```python
from build123d import *

# Parameters (mm, degrees)
F0_W           = 177.8
F0_H           = 101.6
F1_DEPTH       = 3.81
F3_W           = 114.3
F3_H           = 4.318
F4_DEPTH       = 3.811
F5_R           = 9.525
F6_DEPTH       = 9.525
F8_W           = 177.8
F8_H           = 101.6
F8_W_2         = 170.18
F8_H_2         = 93.98
F9_DEPTH       = 7.62
F10_R          = 3.556
F11_DEPTH      = 9.526
F11_DEPTH_BACK = 3.811
F7_W           = 177.8
F7_H           = 3.175
F13_DEPTH      = 7.62
F2_R           = 3.556
F14_DEPTH      = 3.811
F12_R          = 2.667
F15_DEPTH      = 3.811


with BuildPart() as f1:
    # F0 (on Top) → F1 (new body)
    with BuildSketch(Plane.XY):
        with Locations((88.9, 50.8)):
            Rectangle(F0_W, F0_H)
    extrude(amount=F1_DEPTH)

    # F3 (on Top) → F4 (cut, through all)
    with BuildSketch(Plane.XY):
        with Locations((88.9, 88.9)):
            Rectangle(F3_W, F3_H)
        with Locations((88.9, 12.7)):
            Rectangle(F3_W, F3_H)
    extrude(amount=F4_DEPTH, mode=Mode.SUBTRACT)

    # F5 (on Top) → F6 (join)
    with BuildSketch(Plane.XY):
        with Locations((12.7, 50.8)):
            Circle(F5_R)
        with Locations((12.7, 90.805)):
            Circle(F5_R)
        with Locations((12.7, 10.795)):
            Circle(F5_R)
        with Locations((165.1, 90.805)):
            Circle(F5_R)
        with Locations((165.1, 50.8)):
            Circle(F5_R)
        with Locations((165.1, 10.795)):
            Circle(F5_R)
    extrude(amount=-F6_DEPTH)

    # F8 (on Top) → F9 (join)
    with BuildSketch(Plane.XY):
        with Locations((88.9, 50.8)):
            Rectangle(F8_W, F8_H)
        with Locations((88.9, 50.8)):
            Rectangle(F8_W_2, F8_H_2, mode=Mode.SUBTRACT)
    extrude(amount=-F9_DEPTH)

    # F10 (on Top) → F11 (cut, two sides)
    with BuildSketch(Plane.XY) as f11_sk:
        with Locations((165.1, 50.8)):
            Circle(F10_R)
        with Locations((165.1, 90.805)):
            Circle(F10_R)
        with Locations((12.7, 10.795)):
            Circle(F10_R)
        with Locations((12.7, 50.8)):
            Circle(F10_R)
        with Locations((12.7, 90.805)):
            Circle(F10_R)
        with Locations((165.1, 10.795)):
            Circle(F10_R)
    extrude(amount=-F11_DEPTH, mode=Mode.SUBTRACT)
    extrude(f11_sk.sketch, amount=F11_DEPTH_BACK, mode=Mode.SUBTRACT)

    # F7 (on Top) → F13 (join)
    with BuildSketch(Plane.XY):
        with Locations((88.9, 42.8625)):
            Rectangle(F7_W, F7_H)
        with Locations((88.9, 58.7375)):
            Rectangle(F7_W, F7_H)
    extrude(amount=-F13_DEPTH)

    # F2 (on Top) → F14 (cut, through all)
    with BuildSketch(Plane.XY):
        with Locations((22.225, 69.85)):
            Circle(F2_R)
        with Locations((22.225, 31.75)):
            Circle(F2_R)
        with Locations((155.575, 69.85)):
            Circle(F2_R)
        with Locations((155.575, 31.75)):
            Circle(F2_R)
    extrude(amount=F14_DEPTH, mode=Mode.SUBTRACT)

    # F12 (on Top) → F15 (cut, through all)
    with BuildSketch(Plane.XY):
        with Locations((31.75, 50.8)):
            Circle(F12_R)
        with Locations((88.9, 50.8)):
            Circle(F12_R)
        with Locations((146.05, 50.8)):
            Circle(F12_R)
        with Locations((9.525, 25.4)):
            Circle(F12_R)
        with Locations((9.525, 76.2)):
            Circle(F12_R)
        with Locations((168.275, 25.4)):
            Circle(F12_R)
        with Locations((168.275, 76.2)):
            Circle(F12_R)
        with Locations((69.85, 50.8)):
            Circle(F12_R)
        with Locations((107.95, 50.8)):
            Circle(F12_R)
        with Locations((50.8, 50.6974235177)):
            Circle(F12_R)
        with Locations((127, 50.6266094744)):
            Circle(F12_R)
    extrude(amount=F15_DEPTH, mode=Mode.SUBTRACT)


solid = f1.part
```
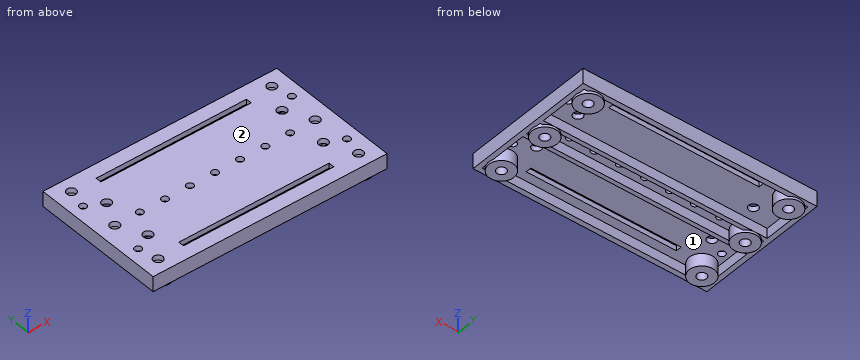
Geometry check sheet. Reference: the model listing, model coordinates, mm. Face numbers are marked on the shaded views. Coordinates: 2 decimals unless noted, no trailing zeros. Order: outer loops, then holes, each group sorted by start corner. A loop starts at its lowest first (then second) coordinate and runs counter-clockwise, first axis right, second up.
Q1. Depth check by flat-ended pin: pin 1 Ø6.5 at (x, y) = (165.1, 10.795) entering from +Z; pin 2 Ø1.5 at (x, y) = (120.5, 23) entering from -Z. Enter the tip coordinate at first touch or a pass-through.
Reply:
pin 1: passes through
pin 2: stops at z = 0
Q2. Sectioned sample at B-B on y = 69.85. Record the cut outline in (x, z), and give its area (3 significant figures).
Reply:
outline: (0, -7.62) - (3.81, -7.62) - (3.81, 0) - (18.67, 0) - (18.67, 3.81) - (0, 3.81) - close; (25.78, 0) - (152.02, 0) - (152.02, 3.81) - (25.78, 3.81) - close; (159.13, 0) - (173.99, 0) - (173.99, -7.62) - (177.8, -7.62) - (177.8, 3.81) - (159.13, 3.81) - close
area: 681 mm2
Q3. Sectioned sample at C-C on z = -2.25. Give the number of separate pieces and of enclosed holes in the cut face, and give its area (3 significant figures).
Reply:
separate pieces: 1
enclosed holes: 17
area: 4,390 mm2
Q4. Draft check along X on the marked faces 1 and 2. Enter one of: released by +X, released by -X, zero draft, split by the parting line, or undercut.
Reply:
face 1: undercut
face 2: zero draft
Q5. Sectioned sample at A-A on x = 127. Record the cut outline in (y, z) (3 decimals).
Reply:
outline: (0, -7.62) - (3.81, -7.62) - (3.81, 0) - (10.541, 0) - (10.541, 3.81) - (0, 3.81) - close; (14.859, 0) - (41.275, 0) - (41.275, -7.62) - (44.45, -7.62) - (44.45, 0) - (47.96, 0) - (47.96, 3.81) - (14.859, 3.81) - close; (53.294, 0) - (57.15, 0) - (57.15, -7.62) - (60.325, -7.62) - (60.325, 0) - (86.741, 0) - (86.741, 3.81) - (53.294, 3.81) - close; (91.059, 0) - (97.79, 0) - (97.79, -7.62) - (101.6, -7.62) - (101.6, 3.81) - (91.059, 3.81) - close
Q6. Thickness scan on probe 1 along Y at (x, z) = (12.5, -0.5) (3 decimals); probe 2 along X at (y, z) = (25.4, 2.65); probe 3 along Y at (x, z) = (151, -2.5) (3 decimals). Record the ranges inside material, lowest first.
Reply:
probe 1: y = 0 to 7.245, 14.345 to 20.318, 41.275 to 47.25, 54.35 to 60.325, 81.282 to 87.255, 94.355 to 101.6
probe 2: x = 0 to 6.86, 12.19 to 165.61, 170.94 to 177.8
probe 3: y = 0 to 3.81, 41.275 to 44.45, 57.15 to 60.325, 97.79 to 101.6
